Autodesk Inventor part; units mm, degrees
ref_plane "YZ Plane" through (0, 0, 0) normal (1, 0, 0) x (0, 1, 0)
ref_plane "XZ Plane" through (0, 0, 0) normal (0, 1, 0) x (-1, 0, 0)
ref_plane "XY Plane" through (0, 0, 0) normal (0, 0, 1) x (1, 0, 0)
ref_plane "Work Plane1" through (0, 0, 0) normal (0, 0, 1) x (1, 0, 0)
sketch "Sketch1" plane through (0, 0, 0) normal (0, 0, 1) x (1, 0, 0)
  line L0 (0, 750) -> (7, 750)
  line L1 (7, 750) -> (7, 1000)
  line L2 (0, 1000) -> (7, 1000)
  line L3 (0, 750) -> (0, 1000)
  line L4 (13, 750) -> (20, 750)
  line L5 (20, 750) -> (20, 1000)
  line L6 (13, 1000) -> (20, 1000)
  line L7 (13, 750) -> (13, 1000)
  line L8 (0, 1000) -> (20, 1000)
  line L9 (20, 1000) -> (20, 983)
  line L10 (20, 983) -> (0, 983)
  line L11 (0, 983) -> (0, 1000)
  line L12 (10, 1000) -> (10, 983) construction
  circle A0 centre (10, 991.5) radius 4.5 construction
  line L13 (0, 985.5) -> (20, 985.5) construction
  point P0 (0, 0)
  point P1 (5.25, 985.5)
  point P2 (14.75, 985.5)
  point P3 (0, 983)
  dimension "d0" = 9
  dimension "d3" = 9.5
  dimension "d4" = 2.5
  dimension "d5" = 17
extrude "Extrusion1" add sketch "Sketch1" along normal blind 5 contours L3 L2 L1 L10 | L1 L8 L7 L10 | L7 L6 L5 L10
hole "Hole1" at (5.25, 985.5, 0) at (14.75, 985.5, 0) direction (0, 0, 1) diameter 2.4 end through all
hole "Hole2" at (10, 991.5, 0) direction (0, 0, 1) diameter 4.5 end through all
sketch "Sketch2" plane through (0, 0, 0) normal (0, 0, -1) x (-1, 0, 0)
  circle A0 centre (-14.75, 985.5) radius 1.2
  circle A1 centre (-5.25, 985.5) radius 1.2
  line L0 (-12.75, 984.3453) -> (-14.75, 983.1906)
  line L1 (-14.75, 983.1906) -> (-16.75, 984.3453)
  line L2 (-16.75, 984.3453) -> (-16.75, 986.6547)
  line L3 (-16.75, 986.6547) -> (-14.75, 987.8094)
  line L4 (-14.75, 987.8094) -> (-12.75, 986.6547)
  line L5 (-12.75, 986.6547) -> (-12.75, 984.3453)
  line L6 (-7.25, 984.3453) -> (-7.25, 986.6547)
  line L7 (-7.25, 986.6547) -> (-5.25, 987.8094)
  line L8 (-5.25, 987.8094) -> (-3.25, 986.6547)
  line L9 (-3.25, 986.6547) -> (-3.25, 984.3453)
  line L10 (-3.25, 984.3453) -> (-5.25, 983.1906)
  line L11 (-5.25, 983.1906) -> (-7.25, 984.3453)
  line L12 (-20, 983) -> (-20, 1000)
  point P0 (0, 0)
  dimension "d22" = 4
extrude "Extrusion2" cut sketch "Sketch2" against normal blind 2
properties part number "ender"
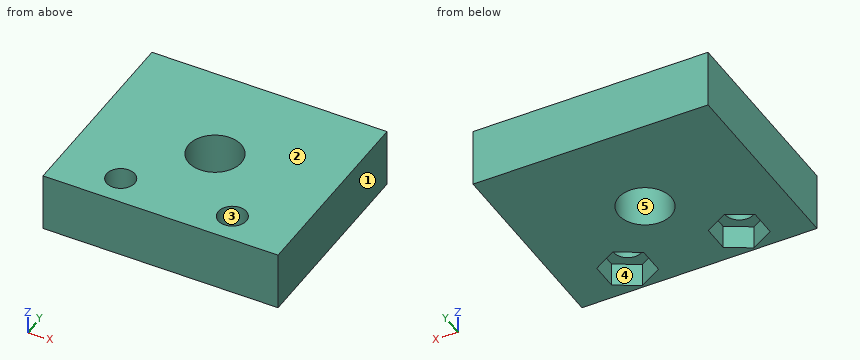
Could you check a few things on this model? Use its own coordinates, in mm. Face numbers are marked on the shaded views. A direction names the side the tool comes from. Give positions to 0.01 mm unless a question says otherwise; leave off trailing zeros. Write each loop counter-clockwise with the first axis right and the second up, starting at its lowest first coordinate (ties: lowest second). Pieces come first, ordered by that corner, then holes. Notation, with made-up numbers: (30, -28) -> (82, -28) arc R13 cw to (82, -17) -> close; hole circle Ø10 at (-16.5, 3). An arc over 180 degrees is marked (long way). Write each question's results on one line, items separated by ' | '. Start each with the question number.
Q1. Which directions (+Z, -Z, +X, -X, +Y, -Y) give clear straight access to the entire face, cutting with the end or side of a thin tool? Please do the marked faces 4 and 5.
Q2. I'm going to push flat-ended pins straight in: pin 1 Ø2 at (x, y) = (14.75, 985.5) entering from -Z; pin 2 Ø1.2 at (x, y) = (15, 984.5) entering from -Z. Where does each tip first touch, or does it pass through?
Q3. Suppose I cut it at A-A, the plane y = 991.5. List the corners of the cut face in (x, z) for me, and give its area (3 significant figures).
Q4. Suppose I cut it at D-D, the plane y = 986.25. List the corners of the cut face in (x, z) for me, and give its area (3 significant figures).
Q5. I need wall thicknesses on probe 1 along X at (y, z) = (985.5, 3.4); probe 2 along X at (y, z) = (991.5, 3.65); probe 3 along Y at (x, z) = (5.25, 4.05). Which ranges of each line are inside material? Lowest first, please.
Q6. Suppose I cut it at C-C, the plane x = 6. List the corners of the cut face in (y, z) for me, and give its area (3 significant figures).
Q7. We'd pull the mould along X, two halves only. Please class the marked faces 1, 2 and 3: +X half, -X half, draft (parallel to the pull), parting line (faces both ways), or undercut.
Q8. Suppose I cut it at B-B, the plane z = 3.05. List the corners of the cut face in (x, y) for me.
Outcome:
1) face 4: -Z | face 5: +Z, -Z
2) pin 1: through | pin 2: z = 2
3) outline: (0, 0) -> (7.75, 0) -> (7.75, 5) -> (0, 5) -> close; (12.25, 0) -> (20, 0) -> (20, 5) -> (12.25, 5) -> close | area: 77.5 mm2
4) outline: (0, 0) -> (3.25, 0) -> (3.25, 2) -> (4.31, 2) -> (4.31, 5) -> (0, 5) -> close; (6.19, 2) -> (7.25, 2) -> (7.25, 0) -> (12.75, 0) -> (12.75, 2) -> (13.81, 2) -> (13.81, 5) -> (6.19, 5) -> close; (15.69, 2) -> (16.75, 2) -> (16.75, 0) -> (20, 0) -> (20, 5) -> (15.69, 5) -> close | area: 72.8 mm2
5) probe 1: 0 to 4.05, 6.45 to 13.55, 15.95 to 20 | probe 2: 0 to 7.75, 12.25 to 20 | probe 3: 983 to 984.3, 986.7 to 1000
6) outline: (983, 0) -> (983.62, 0) -> (983.62, 2) -> (984.56, 2) -> (984.56, 5) -> (983, 5) -> close; (986.44, 2) -> (987.38, 2) -> (987.38, 0) -> (1000, 0) -> (1000, 5) -> (986.44, 5) -> close | area: 71.9 mm2
7) face 1: +X half | face 2: draft | face 3: undercut
8) outline: (0, 983) -> (20, 983) -> (20, 1000) -> (0, 1000) -> close; hole circle Ø2.4 at (5.25, 985.5); hole circle Ø4.5 at (10, 991.5); hole circle Ø2.4 at (14.75, 985.5)
